Read the model definition and answer for the solid it produces. Units are mm, in the model's axes. Round coordinates to 2 decimals unless told otherwise and drop trailing zeros. Write each loop counter-clockwise with the first axis right and the second up, starting at its lowest first coordinate (ties: lowest second). Pieces come first, ordered by that corner, then holes. Notation, with made-up numbers: (4, -14.5) - (13, -14.5) arc R18 ccw to (13, 10.5) - close; hole circle Ø10 at (-13.5, 32.25). An arc over 180 degrees is marked (long way). One line per item, written item: value. Start each with the question number.
(1) Find the intervals of material crossed by L1, parallel to Z at x = -3, y = 24; L2, parallel to X at y = 76.5, z = 2; L3, parallel to X at y = 79, z = 3.6, in increasing order.
(2) A cutting plane is placed at D-D, the plane x = 17. Determine the outline of the cut face in (y, z), plus the area to 3 significant figures.
(3) A cutting plane is placed at B-B, the plane z = 1.95. Determine the outline of the cut face in (x, y).
(4) A cutting plane is placed at C-C, the plane y = 42.5. Determine the outline of the cut face in (x, z), plus the area to 3 significant figures.
(5) Flat-ended cylindrical pins translate along their axes: pin 1 Ø0.6 at (y, z) = (47, 1.5) entering from -X; pin 2 Ø2 at (y, z) = (74, 3) entering from +X. Find the tip coordinate at first contact, or state that the pin passes through.
(6) A cutting plane is placed at A-A, the plane x = 9.5. Determine the outline of the cut face in (y, z).
from build123d import *

# Parameters (mm, degrees)
EXTRUDE_1_DEPTH          = 4
CUT_EXTRUDE_1_DEPTH      = 26
CUT_EXTRUDE_1_DEPTH_BACK = 8.085570508
SKETCH_3_W               = 2
SKETCH_3_H               = 50
CUT_EXTRUDE_2_DEPTH      = 12
CUT_EXTRUDE_2_DEPTH_BACK = 8.085570508


with BuildPart() as part:
    # 草图1 → 凸台-拉伸1 (new body)
    with BuildSketch(Plane.XY):
        with BuildLine():
            Line((-0.350516392, 90), (24.649483608, 90))
            ThreePointArc((24.649483608, 90), (17.915567088, 44.973091345), (25, 0))
            Line((25, 0), (0, 0))
            ThreePointArc((0, 0), (-7.084432912, 44.973091345), (-0.350516392, 90))
        make_face()
    extrude(amount=EXTRUDE_1_DEPTH)

    # 草图2 → 切除-拉伸1 (cut, two sides)
    with BuildSketch(Plane(origin=(0, 0, 0), x_dir=(0, 0, -1), z_dir=(1, 0, 0))) as cut_extrude_1_sk:
        Polygon((-4, 90), (0, 71.181479562), (0, 90), align=None)
    extrude(amount=CUT_EXTRUDE_1_DEPTH, mode=Mode.SUBTRACT)
    extrude(cut_extrude_1_sk.sketch, amount=-CUT_EXTRUDE_1_DEPTH_BACK, mode=Mode.SUBTRACT)

    # 草图3 → 切除-拉伸2 (cut, two sides)
    with BuildSketch(Plane(origin=(0, 0, 0), x_dir=(0, 0, -1), z_dir=(1, 0, 0))) as cut_extrude_2_sk:
        with Locations((-2, 45)):
            Rectangle(SKETCH_3_W, SKETCH_3_H)
    extrude(amount=CUT_EXTRUDE_2_DEPTH, mode=Mode.SUBTRACT)
    extrude(cut_extrude_2_sk.sketch, amount=-CUT_EXTRUDE_2_DEPTH_BACK, mode=Mode.SUBTRACT)


solid = part.part
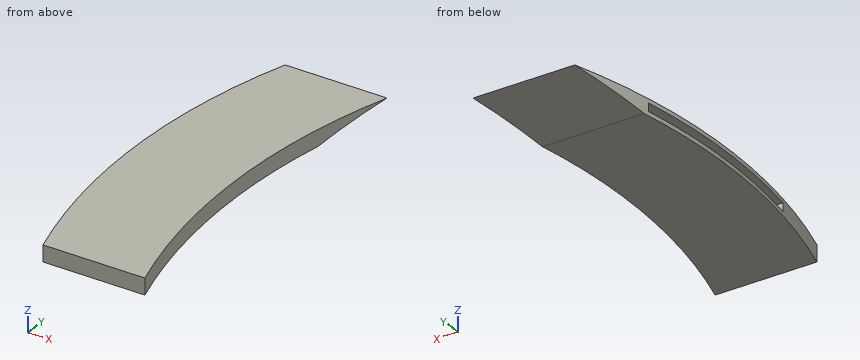
Here are the results:
1. L1: 0 to 1, 3 to 4
1. L2: -3.86 to 21.14
1. L3: -3.31 to 21.69
2. outline: (0, 0) - (71.18, 0) - (90, 4) - (0, 4) - close
2. area: 322 mm²
3. outline: (-5.08, 70) - (12, 70) - (12, 20) - (-4.89, 20) arc R150 ccw to (0, 0) - (25, 0) arc R150 cw to (22.01, 80.36) - (-2.99, 80.36) arc R150 ccw to start
4. outline: (-7.05, 0) - (17.95, 0) - (17.95, 4) - (-7.05, 4) - (-7.05, 3) - (12, 3) - (12, 1) - (-7.05, 1) - close
4. area: 61.9 mm²
5. pin 1: x = 12
5. pin 2: x = 20.83
6. outline: (0, 0) - (71.18, 0) - (90, 4) - (0, 4) - close; hole (20, 1) - (70, 1) - (70, 3) - (20, 3) - close
